The listing builds one solid part. Answer for the finished solid, in the listing's coordinates (mm). Coordinates: 2 decimals unless noted, no trailing zeros. Order: outer loops, then holes, each group sorted by start corner. A loop starts at its lowest first (then second) coordinate and runs counter-clockwise, first axis right, second up. Notation, with made-up numbers: (31, 75.25) -> (83, 75.25) arc R28 ccw to (83, 98.25) -> close; hole circle Ø5 at (-35.5, 50). An arc over 180 degrees is marked (long way). Answer in a Markdown table with one row per item.
```python
from build123d import *

# Parameters (mm, degrees)
F0_R     = 10.795
F1_DEPTH = 1.524


with BuildPart() as f1:
    # F0 (on Front) → F1 (new body)
    with BuildSketch(Plane.XZ):
        with BuildLine():
            ThreePointArc((25.226326, -2.965207), (25.356544, -1.485144), (25.4, 0))
            ThreePointArc((25.4, 0), (14.019199, 21.1807), (-9.924571, 23.380823))
            ThreePointArc((-9.924571, 23.380823), (-15.233656, -20.324757), (25.226326, -2.965207))
        make_face()
        Circle(F0_R, mode=Mode.SUBTRACT)
        with BuildLine():
            ThreePointArc((-9.924571, 23.380823), (14.019199, 21.1807), (25.4, 0))
            ThreePointArc((25.4, 0), (25.356544, -1.485144), (25.226326, -2.965207))
            Line((25.226326, -2.965207), (28.909326, 4.095993))
            Line((28.909326, 4.095993), (28.909326, 8.718793))
            ThreePointArc((28.909326, 8.718793), (29.87646, 11.053659), (32.211326, 12.020793))
            Line((32.211326, 12.020793), (38.307326, 12.020793))
            Line((38.307326, 12.020793), (45.419326, 9.861793))
            Line((45.419326, 9.861793), (45.419326, 28.657793))
            ThreePointArc((45.419326, 28.657793), (47.130409, 32.788711), (51.261326, 34.499793))
            Line((51.261326, 34.499793), (175.721326, 34.499793))
            ThreePointArc((175.721326, 34.499793), (172.001583, 43.480049), (163.021326, 47.199793))
            Line((163.021326, 47.199793), (46.189405, 47.199793))
            Line((46.189405, 47.199793), (-9.924571, 23.380823))
        make_face()
    extrude(amount=F1_DEPTH)


solid = f1.part
```
(1) A cutting plane is placed at B-B, the plane x = 0. Determine the outline of the cut face in (y, z) (3 decimals), then the cut area to 3 significant figures.
Check values:
| item | result |
|---|---|
| outline | (-1.524, -25.4) -> (0, -25.4) -> (0, -10.795) -> (-1.524, -10.795) -> close; (-1.524, 10.795) -> (0, 10.795) -> (0, 27.594) -> (-1.524, 27.594) -> close |
| area | 47.9 mm² |
(2) A cutting plane is placed at C-C, the plane z = 0. Determine the outline of the cut face in (x, y) (3 decimals), then the cut area to 3 significant figures.
Check values:
| item | result |
|---|---|
| outline | (-25.4, -1.524) -> (-10.795, -1.524) -> (-10.795, 0) -> (-25.4, 0) -> close; (10.795, -1.524) -> (26.773, -1.524) -> (26.773, 0) -> (10.795, 0) -> close |
| area | 46.6 mm² |
(3) For a pull along X with two mould halves and no side action, classify faces 1 (the flat face through (27.042, -0.751, 0.516)), 2 (the flat face through (45, -1.524, 22)), 3 (the cylindrical face through (-7.956, -0.751, 7.296)), 4 (the cylindrical face through (29.851, -0.751, 11.028)) as released by +X, released by -X, zero draft, split by the parting line, or undercut.
Check values:
| item | result |
|---|---|
| face 1 | released by +X |
| face 2 | zero draft |
| face 3 | undercut |
| face 4 | undercut |
(4) A cutting plane is placed at D-D, the plane x = 136. Determine the outline of the cut face in (y, z), then the cut area to 3 significant figures.
Check values:
| item | result |
|---|---|
| outline | (-1.52, 34.5) -> (0, 34.5) -> (0, 47.2) -> (-1.52, 47.2) -> close |
| area | 19.4 mm² |
(5) Find the intervals of material crossed by line 1 along Z through (x, y) = (98, -0.35); line 2 along Z through (x, y) = (0, -0.95) (3 decimals); line 3 along X through (y, z) = (-0.5, 7), in increasing order. Write a range as from..to.
Check values:
| item | result |
|---|---|
| line 1 | 34.5..47.2 |
| line 2 | -25.4..-10.795, 10.795..27.594 |
| line 3 | -24.42..-8.22, 8.22..28.91 |
(6) Flat-ended cylindrical pins translate along their axes: pin 1 (0.8 mm diameter, centred on y = -0.5, z = 19.5, fed in from +X); pin 2 (0.5 mm diameter, centred on y = -1, z = 7.5, fed in from +X); pin 3 (13 mm diameter, centred on x = 0, z = 0, fed in from -Y); pin 4 (0.5 mm diameter, centred on x = 35.5, y = -1, fed in from -Z). Find the tip coordinate at first contact, or state that the pin passes through.
Check values:
| item | result |
|---|---|
| pin 1 | x = 45.42 |
| pin 2 | x = 28.91 |
| pin 3 | through |
| pin 4 | z = 12.02 |
(7) A cutting plane is placed at A-A, the plane y = -0.3. Determine the outline of the cut face in (x, z) (3 decimals), then the cut area to 3 significant figures.
Check values:
| item | result |
|---|---|
| outline | (-9.925, 23.381) arc R25.4 ccw (long way) to (25.226, -2.965) -> (28.909, 4.096) -> (28.909, 8.719) arc R3.302 cw to (32.211, 12.021) -> (38.307, 12.021) -> (45.419, 9.862) -> (45.419, 28.658) arc R5.842 cw to (51.261, 34.5) -> (175.721, 34.5) arc R12.7 ccw to (163.021, 47.2) -> (46.189, 47.2) -> close; hole circle Ø21.59 at (0, 0) |
| area | 4,290 mm² |
